The model under review builds one solid part; all positions refer to its coordinate system, in mm. Face numbers are marked on the shaded views. A direction names the side the tool comes from. Coordinates: 2 decimals unless noted, no trailing zeros. Order: outer loops, then holes, each group sorted by start corner. A loop starts at its lowest first (then second) coordinate and runs counter-clockwise, first axis right, second up. Notation, with made-up numbers: (-12.75, 88) -> (19.25, 88) arc R22 ccw to (19.25, 119) -> close; hole circle Ø7 at (54.25, -24). An arc over 180 degrees is marked (long way). Use one line per item in the form item = value.
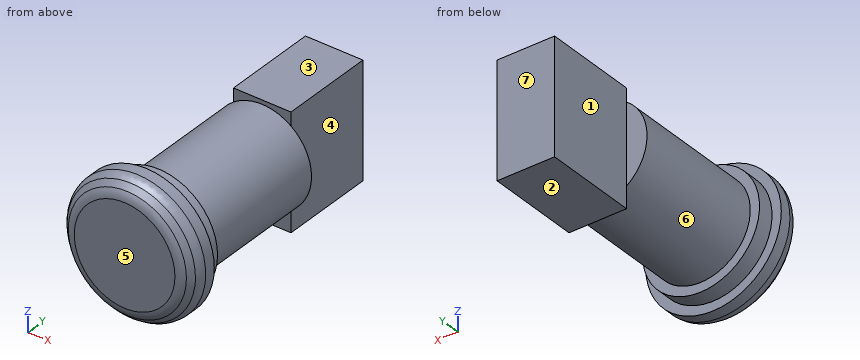
Solid Edge part; units mm, degrees
sketch "Sketch1" plane through (0, 0, 0) normal (0, -1, 0) x (1, 0, 0)
  circle A0 centre (26.4472, -24.7177) radius 16.5
extrude "Protrusion1" add sketch "Sketch1" along normal blind 7
sketch "Sketch2" plane through (0, 0, 0) normal (0, -1, 0) x (1, 0, 0)
  circle A0 centre (26.4472, -24.7177) radius 12
extrude "ExtrudedProtrusion_2" add sketch "Sketch2" against normal blind 37
sketch "Sketch3" plane through (0, 0, 0) normal (0, -1, 0) x (1, 0, 0)
  circle A0 centre (26.4472, -24.7177) radius 14.25
extrude "ExtrudedProtrusion_3" add sketch "Sketch3" against normal blind 4
chamfer "Chamfer_1" distance 3 angle 45 1 edges at (9.9472, -7, -24.7177)
fillet "Round_1" radius 3 2 edges at (26.4472, -4, -41.2177) (26.4472, -7, -38.2177)
sketch "Sketch4" plane through (26.4472, 37, -24.7177) normal (0, 1, 0) x (-1, 0, 0)
  line L0 (7, 13) -> (-7, 13)
  line L1 (-7, 13) -> (-7, -15)
  line L2 (-7, -15) -> (7, -15)
  line L3 (7, -15) -> (7, 13)
extrude "ExtrudedProtrusion_4" add sketch "Sketch4" along normal blind 23
Item 1: To check wall thickness, follow L1, parallel to Z at x = 26.5, y = 21; L2, parallel to Z at x = 33, y = 50.5; L3, parallel to X at y = 53.5, z = -35.5. State the ranges of each line that lie inside material, in increasing order. Write a range as from..to.
Results found:
L1 = -36.72..-12.72
L2 = -39.72..-11.72
L3 = 19.45..33.45
Item 2: We need section B-B (y = 23). Write out the cut boundary in (x, z).
Results found:
outline = circle Ø24 at (26.45, -24.72)
Item 3: We need section A-A (y = 44). Write out the cut boundary in (x, z), plus the area to 3 significant figures.
Results found:
outline = (19.45, -39.72) -> (33.45, -39.72) -> (33.45, -11.72) -> (19.45, -11.72) -> close
area = 392 mm²
Item 4: Draft analysis for pull direction Y (two halves, no side actions). For the marked faces 4, 5, 6 and 7, state which applies: released by +Y, released by -Y, zero draft, split by the parting line, or undercut.
Results found:
face_4 = zero draft
face_5 = released by -Y
face_6 = undercut
face_7 = released by +Y
Item 5: Tool access review of the marked faces 1, 2 and 3: name each direction out of +Z, -Z, +X, -X, +Y, -Y from which nothing blocks a thin tool from reaching the whole face with its end or side.
Results found:
face_1 = +Z, -Z, -X, +Y
face_2 = -Z, +X, -X, +Y
face_3 = +Z, +X, -X, +Y
Item 6: Clearance check with flat-ended pins moving along their axes: pin 1 (4 mm diameter, centred on x = 37.5, y = 32, fed in from -Z); pin 2 (4 mm diameter, centred on y = 1.5, z = -31, fed in from -X); pin 3 (5.5 mm diameter, centred on x = 16.5, z = -25.5, fed in from +Y); pin 4 (5 mm diameter, centred on x = 33.5, z = -35.5, fed in from +Y). State where each tip first meets the part, or that it passes through.
Results found:
pin_1 = -32.59
pin_2 = 10.71
pin_3 = 37
pin_4 = 60
